Autodesk Inventor part; units mm, degrees
ref_plane "YZ Plane" through (0, 0, 0) normal (1, 0, 0) x (0, 1, 0)
ref_plane "XZ Plane" through (0, 0, 0) normal (0, 1, 0) x (-1, 0, 0)
ref_plane "XY Plane" through (0, 0, 0) normal (0, 0, 1) x (1, 0, 0)
sketch "Sketch1" plane through (0, 0, 0) normal (0, 0, 1) x (1, 0, 0)
  line L0 (-76.9591, 41.6961) -> (50.0409, 41.6961)
  line L1 (50.0409, 41.6961) -> (50.0409, 3.5961)
  line L2 (50.0409, 3.5961) -> (-76.9591, 3.5961)
  line L3 (-76.9591, 3.5961) -> (-76.9591, 41.6961)
  circle A0 centre (-28.4591, 22.6461) radius 2.0193
  circle A1 centre (1.5409, 22.6461) radius 2.0193
  circle A2 centre (-64.2591, 22.6461) radius 3.81
  circle A3 centre (37.3409, 22.6461) radius 3.81
  point P0 (0, 0)
  dimension "d0" = 127
  dimension "d1" = 38.1
  dimension "d4" = 4.0386
  dimension "d5" = 4.0386
  dimension "d8" = 7.62
  dimension "d9" = 7.62
extrude "Extrusion1" add sketch "Sketch1" along normal blind 6.35
properties part number "z axis mount"
Input: part model. Units: mm. Frame: model coordinates. Round coordinates to 2 decimals unless told otherwise and drop trailing zeros. Loops run counter-clockwise (first coordinate to the right, second up) from the corner with the lowest first, then second, coordinate; pieces in that order, holes last. Notation, with made-up numbers: M 31.25,-31 L 39.25,-31 A33 cw 39.25,-1 Z; hole C -2.5,89 d9. An arc over 180 degrees is marked long. Answer in a Markdown table with one row per item. Add a question column.
1. Mould query, pull axis X, two halves, no side actions, for faces 1 (the face through (-76.959, 22, 3)), 2 (the face through (1.278, 20.644, 3.131)), 3 (the face through (-27.374, 20.943, 3.131)), 4 (the face through (-14, 23, 6.35)). Classes: released by +X, released by -X, zero draft, split by the parting line, or undercut.
2. Section A-A (z = 1.75). Output: boundary loops of the cut face in (x, y).
3. Ray query, probe 1 along X at (y, z) = (26, 3); probe 2 along Y at (x, z) = (38.5, 1.25); probe 3 along Y at (x, z) = (38, 4.5). Return the intervals inside material, ascending.
Values follow:
| question | item | result |
|---|---|---|
| 1 | face 1 | released by -X |
| 1 | face 2 | undercut |
| 1 | face 3 | undercut |
| 1 | face 4 | zero draft |
| 2 | outline | M -76.96,3.6 L 50.04,3.6 L 50.04,41.7 L -76.96,41.7 Z; hole C -64.26,22.65 d7.62; hole C -28.46,22.65 d4.04; hole C 1.54,22.65 d4.04; hole C 37.34,22.65 d7.62 |
| 3 | probe 1 | -76.96 to -66.07, -62.45 to 35.53, 39.15 to 50.04 |
| 3 | probe 2 | 3.6 to 19.02, 26.28 to 41.7 |
| 3 | probe 3 | 3.6 to 18.89, 26.4 to 41.7 |
